Design review of the part built by this model. Coordinates are the model's own, in mm. Face numbers are marked on the shaded views. A direction names the side the tool comes from. Give positions to 0.01 mm unless a question says otherwise; leave off trailing zeros. Loops run counter-clockwise (first coordinate to the right, second up) from the corner with the lowest first, then second, coordinate; pieces in that order, holes last. Notation, with made-up numbers: (12, -1.75) -> (46, -1.75) arc R27 cw to (46, 29.25) -> close; hole circle Ø8 at (-33, 14.25). An arc over 180 degrees is marked (long way). Use CSV: the item, a comma, the result in double quotes. Start each with the question number.
Item 1: The part is to be moulded in two halves that separate along Y. For the marked faces 3, 4 and 5, say which applies: +Y half, -Y half, draft (parallel to the pull), parting line (faces both ways), or undercut.
Item 2: We need section B-B (z = 18.5). State the section outline as (x, y) points.
Item 3: We need section A-A (z = -11). State the section outline as (x, y) points, plus the area to 3 significant figures.
Item 4: Wall thickness on line 1 along Y through (x, z) = (110, 2); line 2 along X through (y, z) = (-10.25, 7.5); line 3 along Z through (x, y) = (132.5, 7.25): over which ranges is each line inside the solid? List them lowest first. Write a range as from..to.
Item 5: Clearance check with flat-ended pins moving along their axes: pin 1 (10 mm diameter, centred on x = 124, y = 1, fed in from +Z); pin 2 (12 mm diameter, centred on x = 79, y = 5, fed in from +Z). State where each tip first meets the part, or that it passes through.
Item 6: For the marked faces 1 and 2, list the 3-axis set-ups (+Z, -Z, +X, -X, +Y, -Y) from which the entire face can be reached by the end or side of a thin tool; tool diameter is ignored.
Item 7: We need section D-D (x = 130). State the section outline as (y, z) points, plus the area to 3 significant figures.
Item 8: We need section C-C (y = 0). State the section outline as (x, z) points, plus the area to 3 significant figures.
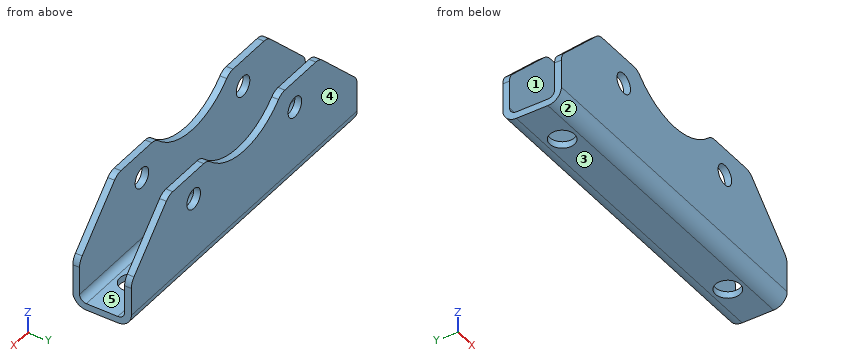
from build123d import *

# Parameters (mm, degrees)
F1_DEPTH = 150
F2_R     = 32.5
F2_R_2   = 4.5
F3_DEPTH = 50
F4_R     = 5.5
F5_DEPTH = 25
F6_SIZE  = 25
F7_R     = 6
F8_DEPTH = 25
F9_R     = 3


with BuildPart() as f1:
    # F0 (on Right) → F1 (new body)
    with BuildSketch(Plane.YZ):
        Polygon((-13, -23), (13, -23), (13, 23), (10, 23), (10, -20), (-10, -20), (-10, 23), (-13, 23), align=None)
    extrude(amount=F1_DEPTH)

    # F2 (on face) → F3 (cut)
    with BuildSketch(Plane.XZ.offset(13)):
        with Locations((75, 44.5)):
            Circle(F2_R)
        with Locations((108.5875721064, 10.9124278936)):
            Circle(F2_R_2)
        with Locations((41.4124278936, 10.9124278936)):
            Circle(F2_R_2)
    extrude(amount=-F3_DEPTH, mode=Mode.SUBTRACT)

    # F4 (on face) → F5 (cut)
    with BuildSketch(Plane.XY.offset(-20)):
        with Locations((20, 0)):
            Circle(F4_R)
        with Locations((130, 0)):
            Circle(F4_R)
    extrude(amount=-F5_DEPTH, mode=Mode.SUBTRACT)

    # F6
    f6_edges = [f1.edges().sort_by_distance(p)[0] for p in [
        (0, 11.5, 23),
        (0, -11.5, 23),
        (150, -11.5, 23),
        (150, 11.5, 23),
    ]]
    chamfer(f6_edges, length=F6_SIZE)

    # F7
    f7_edges = [f1.edges().sort_by_distance(p)[0] for p in [
        (0, -11.5, -2),
        (0, 11.5, -2),
        (25, 11.5, 23),
        (25, -11.5, 23),
        (99.372115, -11.5, 23),
        (50.627885, -11.5, 23),
        (50.627885, 11.5, 23),
        (99.372115, 11.5, 23),
        (125, -11.5, 23),
        (125, 11.5, 23),
        (150, 11.5, -2),
        (150, -11.5, -2),
        (75, -13, -23),
        (75, 13, -23),
    ]]
    fillet(f7_edges, radius=F7_R)

    # F2 (on face) → F8 (cut)
    with BuildSketch(Plane.XZ.offset(13)):
        with Locations((75, 44.5)):
            Circle(F2_R)
        with Locations((108.5875721064, 10.9124278936)):
            Circle(F2_R_2)
        with Locations((41.4124278936, 10.9124278936)):
            Circle(F2_R_2)
    extrude(amount=-F8_DEPTH, mode=Mode.SUBTRACT)

    # F9
    f9_edges = [f1.edges().sort_by_distance(p)[0] for p in [
        (75, 10, -20),
        (75, -10, -20),
    ]]
    fillet(f9_edges, radius=F9_R)


solid = f1.part
Results found:
1,face 3,"draft"
1,face 4,"+Y half"
1,face 5,"undercut"
2,outline,"(20.5, -13) -> (55.5, -13) -> (55.5, -10) -> (20.5, -10) -> close; (20.5, 10) -> (55.5, 10) -> (55.5, 13) -> (20.5, 13) -> close; (94.5, -13) -> (129.5, -13) -> (129.5, -10) -> (94.5, -10) -> close; (94.5, 10) -> (129.5, 10) -> (129.5, 13) -> (94.5, 13) -> close"
3,outline,"(0, -13) -> (150, -13) -> (150, -10) -> (0, -10) -> close; (0, 10) -> (150, 10) -> (150, 13) -> (0, 13) -> close"
3,area,"900 mm²"
4,line 1,"-13..-10, 10..13"
4,line 2,"9.5..38.48, 44.35..105.65, 111.52..140.5"
4,line 3,"-22.99..-19.99"
5,pin 1,"z = -20"
5,pin 2,"z = 12.83"
6,face 1,"+Z, +X, -X"
6,face 2,"-Z, +X, -X, -Y"
7,outline,"(-13, -17) arc R6 ccw to (-7, -23) -> (-5.5, -23) -> (-5.5, -20) -> (-7, -20) arc R3 cw to (-10, -17) -> (-10, 18) -> (-13, 18) -> close; (5.5, -23) -> (7, -23) arc R6 ccw to (13, -17) -> (13, 18) -> (10, 18) -> (10, -17) arc R3 cw to (7, -20) -> (5.5, -20) -> close"
7,area,"261 mm²"
8,outline,"(0, -23) -> (14.5, -23) -> (14.5, -20) -> (0, -20) -> close; (25.5, -23) -> (124.5, -23) -> (124.5, -20) -> (25.5, -20) -> close; (135.5, -23) -> (150, -23) -> (150, -20) -> (135.5, -20) -> close"
8,area,"384 mm²"
